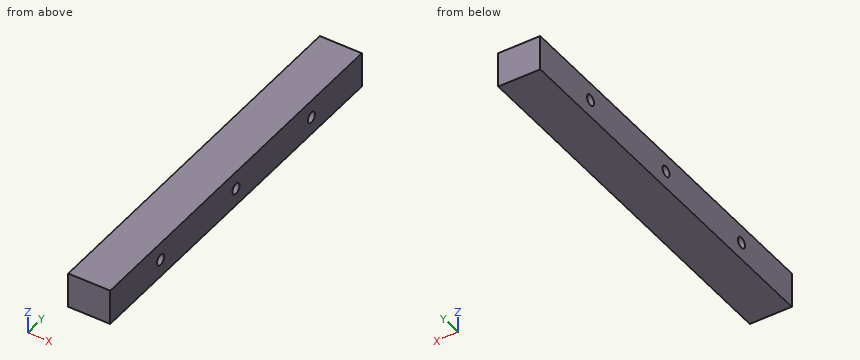
```python
from build123d import *

# Parameters (mm, degrees)
SKETCH1_W           = 13.97
SKETCH1_H           = 127
BOSS_EXTRUDE1_DEPTH = 11.811
SKETCH2_R           = 1.778
CUT_EXTRUDE1_DEPTH  = 14.97


with BuildPart() as part:
    # Sketch1 → Boss-Extrude1 (new body)
    with BuildSketch(Plane.XY):
        with Locations((6.985, 63.5)):
            Rectangle(SKETCH1_W, SKETCH1_H)
    extrude(amount=BOSS_EXTRUDE1_DEPTH)

    # Sketch2 → Cut-Extrude1 (cut, through all)
    with BuildSketch(Plane.ZY):
        with Locations((5.9055, 101.6)):
            Circle(SKETCH2_R)
        with Locations((5.9055, 63.5)):
            Circle(SKETCH2_R)
        with Locations((5.9055, 25.4)):
            Circle(SKETCH2_R)
    extrude(amount=-CUT_EXTRUDE1_DEPTH, mode=Mode.SUBTRACT)


solid = part.part
```
CAD build for the part. Positions are in the model's coordinates, mm. Round coordinates to 2 decimals unless told otherwise and drop trailing zeros. Loops run counter-clockwise (first coordinate to the right, second up) from the corner with the lowest first, then second, coordinate; pieces in that order, holes last. Notation, with made-up numbers: M -3,49 L 52,49 A38 ccw 52,88 Z; hole C -8,-3.5 d11. An arc over 180 degrees is marked long. Use a Markdown table: item, result. Add a question column.
(1) Drill centre lines: line 1 (Y direction, x = 10.5, z = 6); line 2 (Y direction, x = 7, z = 5.25); line 3 (Z direction, x = 8, y = 101.6). Where is each one in solid material? Low to high.
(2) Cut at A-A (y = 101.6). Give the cut face in (x, z), and give its area (3 significant figures).
(3) Cut at B-B (x = 6.25). Give the cut face in (y, z), and give its area (3 significant figures).
Geometry says:
| question | item | result |
|---|---|---|
| 1 | line 1 | y = 0 to 23.62, 27.18 to 61.72, 65.28 to 99.82, 103.38 to 127 |
| 1 | line 2 | y = 0 to 23.75, 27.05 to 61.85, 65.15 to 99.95, 103.25 to 127 |
| 1 | line 3 | z = 0 to 4.13, 7.68 to 11.81 |
| 2 | outline | M 0,0 L 13.97,0 L 13.97,4.13 L 0,4.13 Z; M 0,7.68 L 13.97,7.68 L 13.97,11.81 L 0,11.81 Z |
| 2 | area | 115 mm² |
| 3 | outline | M 0,0 L 127,0 L 127,11.81 L 0,11.81 Z; hole C 25.4,5.91 d3.56; hole C 63.5,5.91 d3.56; hole C 101.6,5.91 d3.56 |
| 3 | area | 1,470 mm² |
